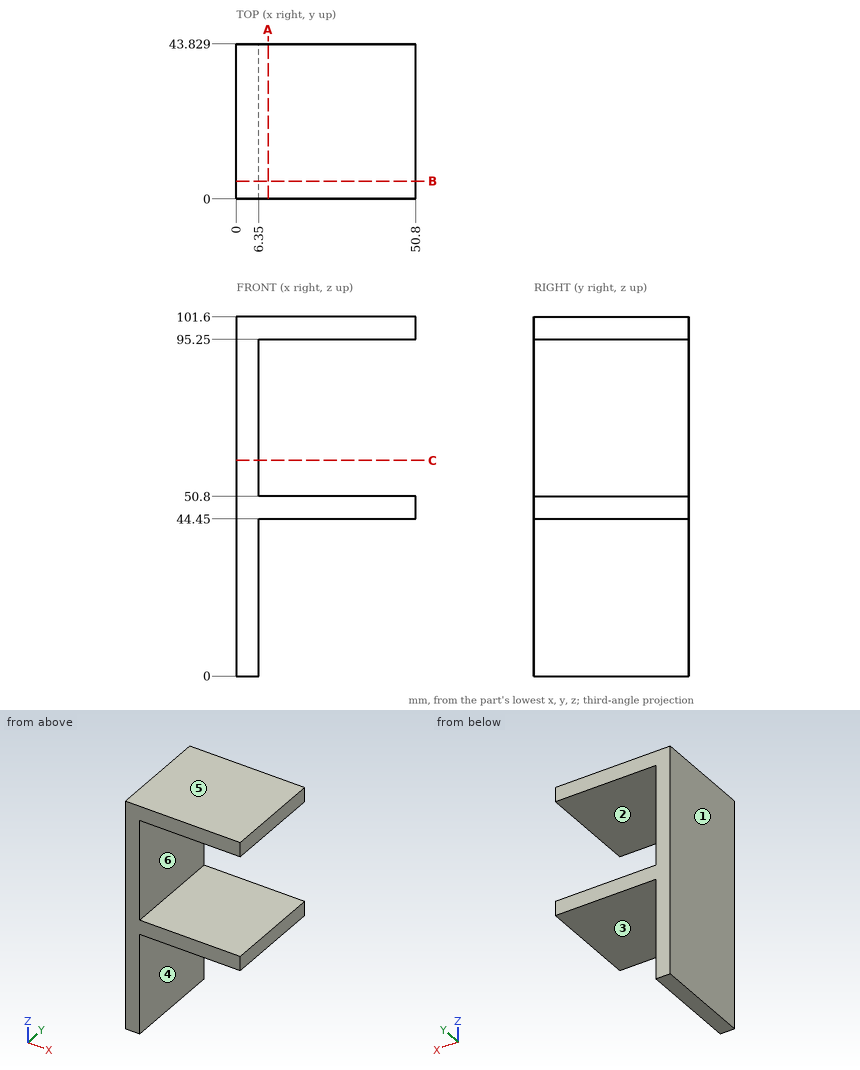
The figure shows three views and two pictorial views of one solid part (mm, origin at its lowest corner). Answer the questions. A direction names the side the tool comes from. Give positions to 0.01 mm unless a question says otherwise; leave off trailing zeros. Write each loop counter-clockwise with the first axis right and the second up, starting at its lowest first coordinate (ties: lowest second). Pieces come first, ordered by that corner, then holes. Notation, with made-up numbers: (-18.5, -6.5) -> (-2.5, -6.5) arc R12 cw to (-2.5, 2.5) -> close; hole circle Ø10 at (87, -28). An arc over 180 degrees is marked (long way). Answer as a JSON object with one key per item and string values.
1) Section A-A on x = 9 is taken. Write down the section's boundary in (y, z).
Findings below:
{"outline": "(0, 44.45) -> (43.83, 44.45) -> (43.83, 50.8) -> (0, 50.8) -> close; (0, 95.25) -> (43.83, 95.25) -> (43.83, 101.6) -> (0, 101.6) -> close"}
2) Straight lines are drawn through the part: probe 1 along Z at (x, y) = (23, 3.5); probe 2 along X at (y, z) = (34, 11). For each, find the intervals that lie inside material, in ascending order. Write a range as from..to.
Findings below:
{"probe 1": "z = 44.45..50.8, 95.25..101.6", "probe 2": "x = 0..6.35"}
3) Flat-ended cylindrical pins translate along their axes: pin 1 Ø13 at (y, z) = (15.5, 12.5) entering from +X; pin 2 Ø1 at (x, y) = (24, 35) entering from -Z. Find the tip coordinate at first contact, or state that the pin passes through.
Findings below:
{"pin 1": "stops at x = 6.35", "pin 2": "stops at z = 44.45"}
4) Section C-C on z = 61 is taken. Write down the section's boundary in (x, y).
Findings below:
{"outline": "(0, 0) -> (6.35, 0) -> (6.35, 43.83) -> (0, 43.83) -> close"}
5) Section B-B on y = 5 is taken. Write down the section's boundary in (x, z), then the cut area to 3 significant figures.
Findings below:
{"outline": "(0, 0) -> (6.35, 0) -> (6.35, 44.45) -> (50.8, 44.45) -> (50.8, 50.8) -> (6.35, 50.8) -> (6.35, 95.25) -> (50.8, 95.25) -> (50.8, 101.6) -> (0, 101.6) -> close", "area": "1,210 mm^2"}
6) A tool of negligible diameter and unlimited length cuts with its end or side. For the marked faces 1, 2 and 3, from which of +Z, -Z, +X, -X, +Y, -Y can it reach the whole face along a straight path? Write none if from no direction.
Findings below:
{"face 1": "+Z, -Z, -X, +Y, -Y", "face 2": "+X, +Y, -Y", "face 3": "-Z, +X, +Y, -Y"}
7) For a pull along Z with two mould halves and no side action, classify the marked faces 4, 5 and 6 as pulls with the +Z half, pulls with the -Z half, needs draft (parallel to the pull), parting line crosses it, or undercut.
Findings below:
{"face 4": "needs draft", "face 5": "pulls with the +Z half", "face 6": "undercut"}
